from build123d import *

# Parameters (mm, degrees)
BASPROSKE_W     = 5
BASPROSKE_H     = 17.5
TOOTHCUT_DEPTH  = 26.248762346
TEETHCUTS_COUNT = 12
TEETHCUTS_ANGLE = 330
BORSKE_R        = 4
BORE_DEPTH      = 50.0000508
EXTRUDE_1_DEPTH = 5
SKETCH_3_R      = 5.787483523
SKETCH_3_R_2    = 1.65
EXTRUDE_2_DEPTH = 5


with BuildPart() as part:
    # BasProSke → Base-Revolve (revolve)
    with BuildSketch(Plane(origin=(0, 0, 0), x_dir=(1, 0, 0), z_dir=(0, 1, 0)), mode=Mode.PRIVATE) as base_revolve_sk:
        with Locations((2.5, 8.75)):
            Rectangle(BASPROSKE_W, BASPROSKE_H)
    revolve(base_revolve_sk.sketch.rotate(Axis((-10, 0, 0), (1, 0, 0)), 180), axis=Axis((-10, 0, 0), (1, 0, 0)))

    # TooCutSke → ToothCut (cut, through all)
    with BuildSketch(Plane(origin=(0, 0, 0), x_dir=(0, 0, -1), z_dir=(1, 0, 0))):
        with BuildLine():
            ThreePointArc((1.394381134, 11.791843675), (0, 11.874), (-1.394381134, 11.791843675))
            ThreePointArc((-1.394381134, 11.791843675), (-2.068078374, 14.771857381), (-4.121860996, 17.033787221))
            ThreePointArc((-4.121860996, 17.033787221), (0, 17.5254), (4.121860996, 17.033787221))
            ThreePointArc((4.121860996, 17.033787221), (2.068078374, 14.771857381), (1.394381134, 11.791843675))
        make_face()
    toothcut = extrude(amount=TOOTHCUT_DEPTH, mode=Mode.SUBTRACT)

    # TeethCuts: ToothCut ×12 about axis
    teethcuts_axis = Axis((-10, 0, 0), (1, 0, 0))
    for i in range(1, TEETHCUTS_COUNT):
        add(toothcut.rotate(teethcuts_axis, i * TEETHCUTS_ANGLE / (TEETHCUTS_COUNT - 1)), mode=Mode.SUBTRACT)

    # BorSke → Bore (cut, symmetric)
    with BuildSketch(Plane(origin=(0, 0, 0), x_dir=(0, 0, -1), z_dir=(1, 0, 0))):
        with Locations(Location((0, 0, 0), (0, 0, 180))):
            Circle(BORSKE_R)
    extrude(amount=BORE_DEPTH, both=True, mode=Mode.SUBTRACT)

    # 草图2 → 凸台-拉伸1 (add)
    with BuildSketch(Plane(origin=(5, 0, 0), x_dir=(0, 0, -1), z_dir=(1, 0, 0))):
        Polygon((0, 11.874), (-5.937, 10.283185645), (-10.595742812, 27.669850518), (-4.658742812, 29.260664873), align=None)
    extrude(amount=-EXTRUDE_1_DEPTH)

    # 草图3 → 凸台-拉伸2 (add)
    with BuildSketch(Plane(origin=(5, 0, 0), x_dir=(0, 0, -1), z_dir=(1, 0, 0))):
        Circle(SKETCH_3_R)
        Circle(SKETCH_3_R_2, mode=Mode.SUBTRACT)
    extrude(amount=-EXTRUDE_2_DEPTH)


solid = part.part
Work out the finished part from the listing and answer in its coordinate system (mm). Give positions to 0.01 mm unless a question says otherwise; leave off trailing zeros. Loops run counter-clockwise (first coordinate to the right, second up) from the corner with the lowest first, then second, coordinate; pieces in that order, holes last. Notation, with made-up numbers: (-14, 53.25) - (34, 53.25) arc R16 cw to (34, 57.25) - close; hole circle Ø1 at (32.5, 51.5). An arc over 180 degrees is marked (long way). Answer in a Markdown table with one row per item.
(1) Section C-C (z = -6.5) is taken. Give the vertices of the cut face in (x, y).
Results list:
| item | result |
|---|---|
| outline | (0, -9.94) - (5, -9.94) - (5, 9.94) - (0, 9.94) - close |
(2) Flat-ended cylindrical pins translate along their axes: pin 1 Ø10 at (y, z) = (-2.5, 7) entering from -X; pin 2 Ø3 at (x, z) = (1.5, 1) entering from -Y. Find the tip coordinate at first contact, or state that the pin passes through.
Results list:
| item | result |
|---|---|
| pin 1 | stops at x = 0 |
| pin 2 | stops at y = -15.48 |
(3) For a pull along Y with two mould halves and no side action, classify faces 1 (the face through (2.54, 4.54, 16.9)), 2 (the face through (2.46, 9.13, -11.73)), 3 (the face through (2.535, -16.905, -4.523)) as pulls with the +Y half, pulls with the -Y half, needs draft (parallel to the pull), parting line crosses it, or undercut.
Results list:
| item | result |
|---|---|
| face 1 | pulls with the +Y half |
| face 2 | undercut |
| face 3 | pulls with the -Y half |
(4) Section B-B (z = 10) is taken. Give the vertices of the cut face in (x, y), and give its area (3 significant figures).
Results list:
| item | result |
|---|---|
| outline | (0, -12.2) - (5, -12.2) - (5, -7.39) - (0, -7.39) - close; (0, -6.4) - (5, -6.4) - (5, 6.4) - (0, 6.4) - close; (0, 7.39) - (5, 7.39) - (5, 12.2) - (0, 12.2) - close; (0, 25.45) - (5, 25.45) - (5, 27.83) - (0, 27.83) - close |
| area | 124 mm² |
(5) Section D-D (y = 26) is taken. Give the vertices of the cut face in (x, z), and give its area (3 significant figures).
Results list:
| item | result |
|---|---|
| outline | (0, 3.79) - (5, 3.79) - (5, 10.15) - (0, 10.15) - close |
| area | 31.8 mm² |
(6) Section A-A (y = 0) is taken. Give the vertices of the cut face in (x, z).
Results list:
| item | result |
|---|---|
| outline | (0, -11.87) - (5, -11.87) - (5, -1.65) - (0, -1.65) - close; (0, 1.65) - (5, 1.65) - (5, 11.87) - (0, 11.87) - close |
(7) Consider L1, parallel to Z at x = 2.8, y = -12 (3 decimals); L2, parallel to Z at x = 1.3, y = 14; L3, parallel to Y at x = 1.9, z = -11.5. Determine where each line is inside the solid, lowest interval first. Write a range as [from, to].
Results list:
| item | result |
|---|---|
| L1 | z = [-12.686, -9.591], [-5.225, -1.391], [1.391, 5.225], [9.591, 12.686] |
| L2 | z = [-5.6, -1.73], [0.57, 6.93] |
| L3 | y = [-12.63, -8.8], [-5.01, 5.01], [8.8, 12.63] |
